The listing builds one solid part. Answer for the finished solid, in the listing's coordinates (mm). A direction names the side the tool comes from. Give positions to 0.01 mm unless a question says otherwise; leave off trailing zeros. Order: outer loops, then holes, each group sorted by start corner. A loop starts at its lowest first (then second) coordinate and runs counter-clockwise, first axis right, second up. Notation, with made-up numbers: (-23.75, 57.5) - (0.25, 57.5) arc R21 ccw to (0.25, 64.5) - close; hole circle Ø11 at (88, 36.25). An arc over 180 degrees is marked (long way). Answer in a Markdown table with one row per item.
Autodesk Inventor part; units mm, degrees
ref_plane "YZ Plane" through (0, 0, 0) normal (1, 0, 0) x (0, 1, 0)
ref_plane "XZ Plane" through (0, 0, 0) normal (0, 1, 0) x (-1, 0, 0)
ref_plane "XY Plane" through (0, 0, 0) normal (0, 0, 1) x (1, 0, 0)
sketch "Sketch1" plane through (0, 0, 0) normal (0, 0, 1) x (1, 0, 0)
  circle A0 centre (0, 0) radius 57.15
  line L0 (2.4402, 2.5908) -> (2.4402, -2.5908)
  line L1 (-2.4402, -2.5908) -> (-2.4402, 2.5908)
  line L2 (-2.4402, 2.5908) -> (2.4402, -2.5908) construction
  line L3 (2.4402, 2.5908) -> (-2.4402, -2.5908) construction
  arc A1 (2.4402, 2.5908) -> (-2.4402, 2.5908) centre (0, -0.0111) ccw
  arc A2 (-2.4402, -2.5908) -> (2.4402, -2.5908) centre (0, -0.0696) ccw
  dimension "d0" = 114.3
  dimension "d1" = 5.1816
  dimension "d2" = 4.8803
  dimension "d5" = 3.5671
extrude "Extrusion2" add sketch "Sketch1" along normal blind 25.4
properties part number "lazy susan platform"
Item 1: Find section A-A on y = 0. Write down the section's boundary in (x, z).
Answer block:
| item | result |
|---|---|
| outline | (-57.15, 0) - (-2.44, 0) - (-2.44, 25.4) - (-57.15, 25.4) - close; (2.44, 0) - (57.15, 0) - (57.15, 25.4) - (2.44, 25.4) - close |
Item 2: Find section D-D on y = -46. Write down the section's boundary in (x, z).
Answer block:
| item | result |
|---|---|
| outline | (-33.91, 0) - (33.91, 0) - (33.91, 25.4) - (-33.91, 25.4) - close |
Item 3: Determine the mould class of faces 3 (the face through (0.04, -3.58, 12.52)), 4 (the face through (-1, -12, 0)), 5 (the face through (-57.095, -2.513, 12.522)) for opening direction X: pulls with the +X half, pulls with the -X half, needs draft (parallel to the pull), parting line crosses it, or undercut.
Answer block:
| item | result |
|---|---|
| face 3 | undercut |
| face 4 | needs draft |
| face 5 | parting line crosses it |
Item 4: Find section C-C on z = 16. Write down the section's boundary in (x, y), then the cut area to 3 significant figures.
Answer block:
| item | result |
|---|---|
| outline | circle Ø114.3 at (0, 0); hole (-2.44, -2.59) arc R3.51 ccw to (2.44, -2.59) - (2.44, 2.59) arc R3.57 ccw to (-2.44, 2.59) - close |
| area | 10,200 mm² |
Item 5: Each of these flat-tipped pins is pushed along its axis until it touches: P1, Ø12, axis at y = 39, z = 15, coming from the -X side; P2, Ø6, axis at x = -1.5, z = 7.5, coming from the -Y side; P3, Ø1.6, axis at y = 1, z = 11, coming from the -X side. Where does it stop, or does it pass through?
Answer block:
| item | result |
|---|---|
| P1 | x = -46.66 |
| P2 | y = -57.15 |
| P3 | x = -57.15 |
Item 6: Consider line 1 (X direction, y = 2.5, z = 2.25); line 2 (Y direction, x = -47, z = 12.5); line 3 (Y direction, x = -40, z = 4.75). Determine where each line is inside the solid, lowest interval first.
Answer block:
| item | result |
|---|---|
| line 1 | -57.1 to -2.44, 2.44 to 57.1 |
| line 2 | -32.51 to 32.51 |
| line 3 | -40.82 to 40.82 |
Item 7: Which of the six approach directions +Z, -Z, +X, -X, +Y, -Y give full straight-line access (tool end or side, diameter ignored) to faces 1 (the face through (-1, -12, 25.4)), 2 (the face through (-0.038, 3.556, 12.522))?
Answer block:
| item | result |
|---|---|
| face 1 | +Z, +X, -X, +Y, -Y |
| face 2 | +Z, -Z |
Item 8: Find section B-B on x = 0. Write down the section's boundary in (y, z), then the cut area to 3 significant figures.
Answer block:
| item | result |
|---|---|
| outline | (-57.15, 0) - (-3.58, 0) - (-3.58, 25.4) - (-57.15, 25.4) - close; (3.56, 0) - (57.15, 0) - (57.15, 25.4) - (3.56, 25.4) - close |
| area | 2,720 mm² |
